Study the drawing (mm; zero at the part's minimum x, y, z) and answer. Coordinates: 2 decimals unless noted, no trailing zeros. Order: outer loops, then holes, each group sorted by start corner. A loop starts at its lowest first (then second) coordinate and runs counter-clockwise, first axis right, second up. Notation, with made-up numbers: M -24,-7.5 L -19,-7.5 A21 ccw -19,14.5 Z; hole C -21,-36.75 d5. An arc over 180 degrees is marked long. Use a Markdown table: item, result. Add a question column.
1) Find section C-C on y = 5. Write down the section's boundary in (x, z).
2) Find section B-B on y = 12.25. Write down the section's boundary in (x, z), plus the area to 4 significant figures.
3) Find the intervals of material crossed by probe 1 along Y at (x, z) = (15, 96); probe 2 along X at (y, z) = (15, 32.5); probe 3 along X at (y, z) = (10.25, 90.5), in increasing order. Write a range as [from, to].
4) Each of these flat-tipped pins is pushed along its axis until it touches: pin 1 Ø6 at (y, z) = (12.5, 82) entering from +X; pin 2 Ø6 at (y, z) = (5, 69.5) entering from -X; pin 3 Ø2 at (y, z) = (2, 12.5) entering from +X. Where does it stop, or does it pass through?
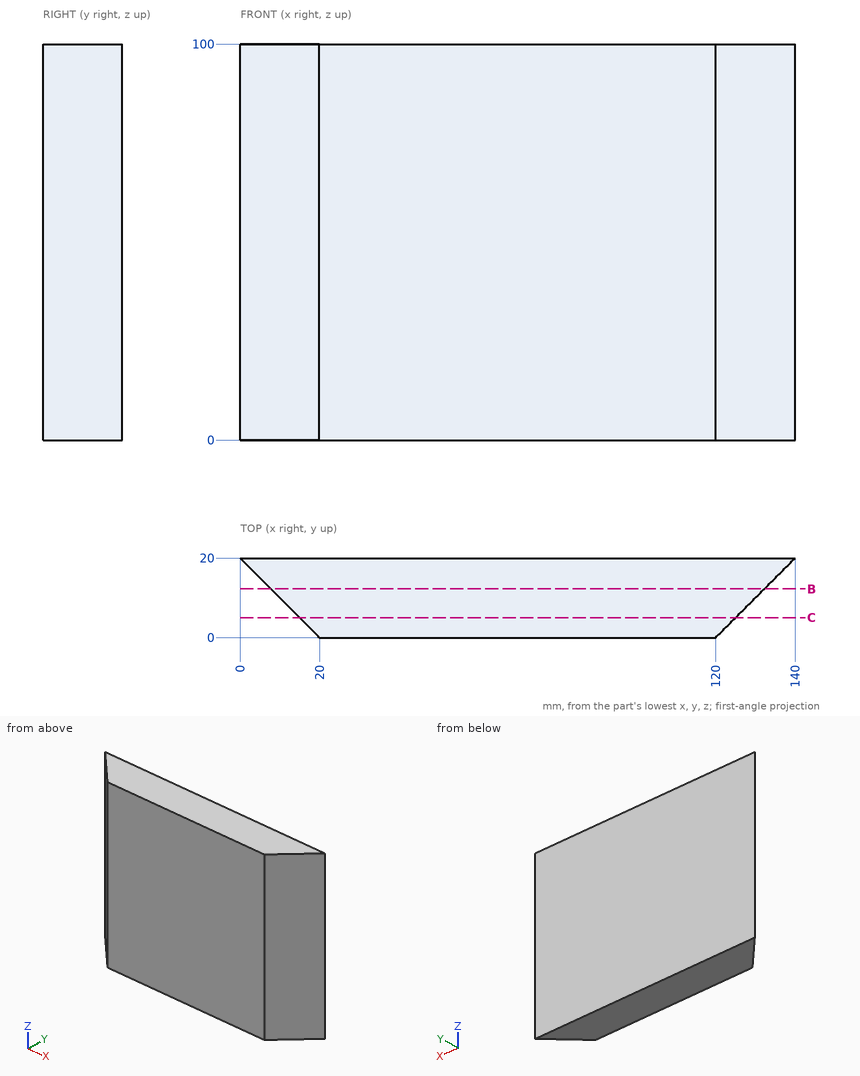
Check result:
| question | item | result |
|---|---|---|
| 1 | outline | M 15,0 L 125,0 L 125,100 L 15,100 Z |
| 2 | outline | M 7.75,0 L 132.25,0 L 132.25,100 L 7.75,100 Z |
| 2 | area | 12,450 mm2 |
| 3 | probe 1 | y = [5, 20] |
| 3 | probe 2 | x = [5, 135] |
| 3 | probe 3 | x = [9.75, 130.25] |
| 4 | pin 1 | stops at x = 135.5 |
| 4 | pin 2 | stops at x = 12 |
| 4 | pin 3 | stops at x = 123 |
